Source: CAD feature listing. Evaluate the final solid. Frame: model axes, mm. Face numbers are marked on the shaded views. A direction names the side the tool comes from. Give positions to 0.01 mm unless a question says otherwise; leave off trailing zeros. Write each loop counter-clockwise with the first axis right and the second up, starting at its lowest first coordinate (ties: lowest second). Pieces come first, ordered by that corner, then holes.
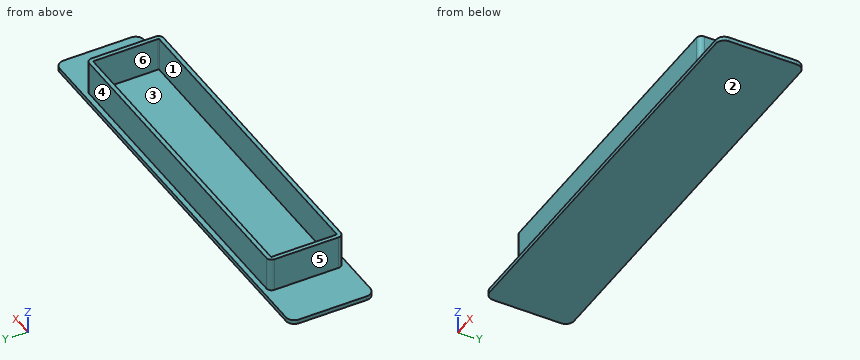
```python
from build123d import *

# Parameters (mm, degrees)
F0_W     = 250
F0_H     = 50
F1_DEPTH = 2.5
F2_W     = 194
F2_H     = 44
F3_DEPTH = 20
F4_R     = 3
F5_T     = -2.5
F6_R     = 5


with BuildPart() as f1:
    # F0 (on Top) → F1 (new body)
    with BuildSketch(Plane.XY):
        with Locations((-100, 25)):
            Rectangle(F0_W, F0_H)
    extrude(amount=F1_DEPTH)

    # F2 (on face) → F3 (join)
    with BuildSketch(Plane.XY.offset(2.5)):
        with Locations((-100, 25)):
            Rectangle(F2_W, F2_H)
    extrude(amount=F3_DEPTH)

    # F4
    f4_edges = [f1.edges().sort_by_distance(p)[0] for p in [
        (-197, 3, 12.5),
        (-3, 3, 12.5),
        (-3, 47, 12.5),
        (-197, 47, 12.5),
    ]]
    fillet(f4_edges, radius=F4_R)

    # F5
    f5_openings = [f1.faces().sort_by_distance(p)[0] for p in [
        (-100, 25, 22.5),
    ]]
    offset(amount=F5_T, openings=f5_openings, kind=Kind.INTERSECTION)

    # F6
    f6_edges = [f1.edges().sort_by_distance(p)[0] for p in [
        (25, 0, 1.25),
        (25, 50, 1.25),
        (-225, 50, 1.25),
        (-225, 0, 1.25),
    ]]
    fillet(f6_edges, radius=F6_R)


solid = f1.part
```
1. Section query A-A (z = 9.5). Return loops of the section in (x, y), plus the area to 3 significant figures.
2. Section query C-C (y = 8.5). Return loops of the section in (x, z), plus the area to 3 significant figures.
3. Access query for the marked faces 5 and 6. Directions: +Z, -Z, +X, -X, +Y, -Y. A direction counts if a zero-diameter tool reaches every point of the face in a straight line with its end or side. Return the directions, or none.
4. Section query D-D (x = 7). Return loops of the section in (y, z).
5. Pin query (flat end, axial travel): P1, Ø6, axis at x = -68, z = 16.5, coming from the +Y side; P2, Ø10, axis at y = 30, z = 12.5, coming from the -X side; P3, Ø2, axis at x = -131, z = 16.5, coming from the -Y side. Return the tip coordinate at first contact, or that it passes through.
6. Section query B-B (x = -38.5). Return loops of the section in (y, z), plus the area to 3 significant figures.
7. Line query: probe 1 along X at (y, z) = (25, 15.5); probe 2 along Y at (x, z) = (-20.5, 12.25); probe 3 along Z at (x, y) = (-111.5, 18.5). Output: solid intervals per line, ascending.
8. Pull-direction query (Y, two-part tool) for the marked faces 1, 2, 3 and 4; classes: pulls with the +Y half, pulls with the -Y half, needs draft (parallel to the pull), parting line crosses it, or undercut.
The answers:
1. outline: (-197, 6) arc R3 ccw to (-194, 3) - (-6, 3) arc R3 ccw to (-3, 6) - (-3, 44) arc R3 ccw to (-6, 47) - (-194, 47) arc R3 ccw to (-197, 44) - close; hole (-194.5, 6) arc R0.5 ccw to (-194, 5.5) - (-6, 5.5) arc R0.5 ccw to (-5.5, 6) - (-5.5, 44) arc R0.5 ccw to (-6, 44.5) - (-194, 44.5) arc R0.5 ccw to (-194.5, 44) - close
1. area: 1,160 mm2
2. outline: (-225, 0) - (25, 0) - (25, 2.5) - (-3, 2.5) - (-3, 22.5) - (-5.5, 22.5) - (-5.5, 2.5) - (-194.5, 2.5) - (-194.5, 22.5) - (-197, 22.5) - (-197, 2.5) - (-225, 2.5) - close
2. area: 725 mm2
3. face 5: +Z, -X, +Y, -Y
3. face 6: +Z
4. outline: (0, 0) - (50, 0) - (50, 2.5) - (0, 2.5) - close
5. P1: stops at y = 47
5. P2: stops at x = -197
5. P3: stops at y = 3
6. outline: (0, 0) - (50, 0) - (50, 2.5) - (47, 2.5) - (47, 22.5) - (44.5, 22.5) - (44.5, 2.5) - (5.5, 2.5) - (5.5, 22.5) - (3, 22.5) - (3, 2.5) - (0, 2.5) - close
6. area: 225 mm2
7. probe 1: x = -197 to -194.5, -5.5 to -3
7. probe 2: y = 3 to 5.5, 44.5 to 47
7. probe 3: z = 0 to 2.5
8. face 1: undercut
8. face 2: needs draft
8. face 3: undercut
8. face 4: pulls with the +Y half
